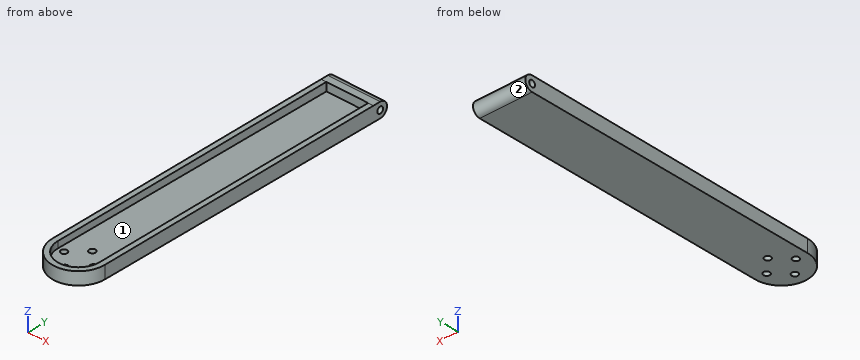
from build123d import *

# Parameters (mm, degrees)
SKETCH_1_R          = 1.5
EXTRUDE_1_DEPTH     = 3
EXTRUDE_3_DEPTH     = 25
SKETCH_4_R          = 1.5
EXTRUDE_5_DEPTH     = 25
CUT_EXTRUDE_1_DEPTH = 25


with BuildPart() as part:
    # 草图1 → 凸台-拉伸1 (new body)
    with BuildSketch(Plane.XY):
        with BuildLine():
            Line((-12.5, -62.82700984), (-12.5, 75.32700984))
            Line((-12.5, 75.32700984), (12.5, 75.32700984))
            Line((12.5, 75.32700984), (12.5, -62.82700984))
            ThreePointArc((12.5, -62.82700984), (0, -75.32700984), (-12.5, -62.82700984))
        make_face()
        with Locations((7, -62.82700984)):
            Circle(SKETCH_1_R, mode=Mode.SUBTRACT)
        with Locations((0, -69.82700984)):
            Circle(SKETCH_1_R, mode=Mode.SUBTRACT)
        with Locations((-7, -62.82700984)):
            Circle(SKETCH_1_R, mode=Mode.SUBTRACT)
        with Locations((0, -55.82700984)):
            Circle(SKETCH_1_R, mode=Mode.SUBTRACT)
    extrude(amount=EXTRUDE_1_DEPTH)

    # 草图3 → 凸台-拉伸3 (add)
    with BuildSketch(Plane.XY.offset(3)):
        with BuildLine():
            Line((10, -62.82700984), (10, 72.82700984))
            Line((10, 72.82700984), (10, 75.32700984))
            Line((10, 75.32700984), (12.5, 75.32700984))
            Line((12.5, 75.32700984), (12.5, -62.82700984))
            ThreePointArc((12.5, -62.82700984), (0, -75.32700984), (-12.5, -62.82700984))
            Line((-12.5, -62.82700984), (-12.5, 75.32700984))
            Line((-12.5, 75.32700984), (-10, 75.32700984))
            Line((-10, 75.32700984), (-10, 72.82700984))
            Line((-10, 72.82700984), (-10, -62.82700984))
            ThreePointArc((-10, -62.82700984), (0, -72.82700984), (10, -62.82700984))
        make_face()
    extrude(amount=EXTRUDE_3_DEPTH)

    # 草图4 → 凸台-拉伸5 (add)
    with BuildSketch(Plane(origin=(12.5, 0, 0), x_dir=(0, 0, -1), z_dir=(1, 0, 0))):
        with BuildLine():
            Line((-3, 75.32700984), (0, 75.32700984))
            Line((0, 75.32700984), (0, 78.791111455))
            ThreePointArc((0, 78.791111455), (-3.511355462, 82.291093034), (-6.999926316, 78.768400651))
            Line((-6.999926316, 78.768400651), (-6.977595346, 75.32700984))
            Line((-6.977595346, 75.32700984), (-3.5, 75.32700984))
            Line((-3.5, 75.32700984), (-3, 75.32700984))
        make_face()
        with Locations((-3.5, 78.791111455)):
            Circle(SKETCH_4_R, mode=Mode.SUBTRACT)
    extrude(amount=-EXTRUDE_5_DEPTH)

    # 草图5 → 切除-拉伸1 (cut)
    with BuildSketch(Plane(origin=(12.5, 0, 0), x_dir=(0, 0, -1), z_dir=(1, 0, 0))):
        Polygon((-6, -75.32700984), (-6.977595346, 75.32700984), (-30.364009186, 75.32700984), (-30.364009186, -75.32700984), align=None)
    extrude(amount=-CUT_EXTRUDE_1_DEPTH, mode=Mode.SUBTRACT)


solid = part.part
Could you check a few things on this model? Use its own coordinates, in mm. Face numbers are marked on the shaded views. Give positions to 0.01 mm unless a question says otherwise; leave off trailing zeros. Loops run counter-clockwise (first coordinate to the right, second up) from the corner with the lowest first, then second, coordinate; pieces in that order, holes last. Notation, with made-up numbers: (-32, 61.5) -> (18, 61.5) arc R10 ccw to (18, 68.5) -> close; hole circle Ø10 at (53.25, 2). An arc over 180 degrees is marked (long way). Return JSON: item names as keys, results as strings.
Item 1: If we section it at B-B on x = 0: List the corners of the cut face in (y, z) for me.
Geometry results:
{"outline": "(-75.33, 0) -> (-71.33, 0) -> (-71.33, 3) -> (-72.83, 3) -> (-72.83, 6.02) -> (-75.33, 6) -> close; (-68.33, 0) -> (-57.33, 0) -> (-57.33, 3) -> (-68.33, 3) -> close; (-54.33, 0) -> (78.79, 0) arc R3.5 ccw (long way) to (78.77, 7) -> (75.33, 6.98) -> (75.33, 3) -> (-54.33, 3) -> close; hole circle Ø3 at (78.79, 3.5)"}
Item 2: We'd pull the mould along X, two halves only. Please class the marked faces 1 and 2: +X half, -X half, draft (parallel to the pull), parting line (faces both ways), or undercut.
Geometry results:
{"face 1": "undercut", "face 2": "draft"}
Item 3: If we section it at C-C on y = -59: List the corners of the cut face in (x, z) for me.
Geometry results:
{"outline": "(-12.5, 0) -> (12.5, 0) -> (12.5, 6.11) -> (10, 6.11) -> (10, 3) -> (-10, 3) -> (-10, 6.11) -> (-12.5, 6.11) -> close"}
Item 4: I need wall thicknesses on L1, parallel to X at y = -56.5, z = 3.25; L2, parallel to Y at x = 6.5, z = 3.75; L3, parallel to Y at x = 0, z = 3.75. Which ranges of each line are inside material? Lowest first, please. Write a range as from..to.
Geometry results:
{"L1": "x = -12.5..-10, 10..12.5", "L2": "y = -73.5..-70.43, 75.33..77.31, 80.27..82.28", "L3": "y = -75.33..-72.83, 75.33..77.31, 80.27..82.28"}
Item 5: If we section it at A-A on x = 7: List the corners of the cut face in (y, z) for me, plus the area to 3 significant figures.
Geometry results:
{"outline": "(-73.18, 0) -> (-64.33, 0) -> (-64.33, 3) -> (-69.97, 3) -> (-69.97, 6.03) -> (-73.18, 6.01) -> close; (-61.33, 0) -> (78.79, 0) arc R3.5 ccw (long way) to (78.77, 7) -> (75.33, 6.98) -> (75.33, 3) -> (-61.33, 3) -> close; hole circle Ø3 at (78.79, 3.5)", "area": "483 mm²"}
Item 6: I'm going to push flat-ended pins straight in: pin 1 (1 mm diameter, centred on x = -2, y = 18.5, fed in from +Z); pin 2 (2.5 mm diameter, centred on x = 0, y = -69.83, fed in from +Z); pin 3 (5 mm diameter, centred on x = 0, y = -55.83, fed in from -Z); pin 4 (3 mm diameter, centred on x = -3, z = 3, fed in from -Y). Where does each tip first touch, or does it pass through?
Geometry results:
{"pin 1": "stops at z = 3", "pin 2": "passes through", "pin 3": "stops at z = 0", "pin 4": "stops at y = -75.24"}
